from build123d import *

# Parameters (mm, degrees)
EXTRUDE_1_DEPTH     = 10
CUT_EXTRUDE_1_REACH = 177.427
SKETCH_2_R          = 2.15
FILLET_1_R          = 0.6


with BuildPart() as part:
    # 草图1 → 凸台-拉伸1 (new body)
    with BuildSketch(Plane(origin=(0, 0, 0), x_dir=(1, 0, 0), z_dir=(0, 1, 0))):
        with BuildLine():
            Line((-19, 0), (19, 0))
            Line((19, 0), (44.854614973, 30.81233028))
            ThreePointArc((44.854614973, 30.81233028), (46.529317931, 33.929104052), (46.82231051, 37.455159084))
            Line((46.82231051, 37.455159084), (33.389549678, 146.856216784))
            ThreePointArc((33.389549678, 146.856216784), (34.753999407, 148.533855984), (36.376927445, 147.104765038))
            ThreePointArc((36.376927445, 147.104765038), (36.892496808, 144.296291333), (37.320815542, 141.473193853))
            Line((37.320815542, 141.473193853), (37.815132232, 139.258398169))
            ThreePointArc((37.815132232, 139.258398169), (37.817176658, 139.245056143), (37.817405692, 139.231560332))
            Line((37.817405692, 139.231560332), (37.557917484, 134.104765038))
            ThreePointArc((37.557917484, 134.104765038), (40.754926912, 130.959847465), (43.503129215, 134.503681536))
            Line((43.503129215, 134.503681536), (43.077003941, 137.813685213))
            Line((43.077003941, 137.813685213), (42.807637334, 138.925557366))
            ThreePointArc((42.807637334, 138.925557366), (42.806315787, 138.931905108), (42.80540838, 138.938325149))
            Line((42.80540838, 138.938325149), (42.129277547, 145.175318139))
            Line((42.129277547, 145.175318139), (41.965181023, 146.44996701))
            ThreePointArc((41.965181023, 146.44996701), (43.130662006, 148.010841711), (44.727999785, 146.895858405))
            Line((44.727999785, 146.895858405), (66.016482503, 37.376109146))
            ThreePointArc((66.016482503, 37.376109146), (66.063066684, 33.817543133), (64.860464706, 30.468019192))
            Line((64.860464706, 30.468019192), (38.23055697, -15.656334008))
            ThreePointArc((38.23055697, -15.656334008), (35.050772773, -18.836118205), (30.707106781, -20))
            Line((30.707106781, -20), (5.707106781, -20))
            ThreePointArc((5.707106781, -20), (5.515765065, -19.961939766), (5.353553391, -19.853553391))
            Line((5.353553391, -19.853553391), (5, -19.5))
            Line((5, -19.5), (-5, -19.5))
            Line((-5, -19.5), (-5.353553391, -19.853553391))
            ThreePointArc((-5.353553391, -19.853553391), (-5.515765065, -19.961939766), (-5.707106781, -20))
            Line((-5.707106781, -20), (-25.399802658, -20))
            ThreePointArc((-25.399802658, -20), (-30.087775174, -18.833058003), (-33.681629288, -15.604582738))
            Line((-33.681629288, -15.604582738), (-64.860464706, 30.468019192))
            ThreePointArc((-64.860464706, 30.468019192), (-66.063066684, 33.817543133), (-66.016482503, 37.376109146))
            Line((-66.016482503, 37.376109146), (-46.829620455, 141.890886738))
            ThreePointArc((-46.829620455, 141.890886738), (-43.465252598, 152.148967586), (-37.480163066, 161.13372674))
            ThreePointArc((-37.480163066, 161.13372674), (-33.620696298, 161.680216975), (-32.479267504, 157.953116813))
            ThreePointArc((-32.479267504, 157.953116813), (-35.579400499, 146.14570295), (-34.973851142, 133.953116813))
            Line((-34.973851142, 133.953116813), (-47.176674229, 34.569098196))
            ThreePointArc((-47.176674229, 34.569098196), (-47.109221395, 33.75732882), (-46.723670812, 33.03978429))
            Line((-46.723670812, 33.03978429), (-19, 0))
        make_face()
    extrude(amount=EXTRUDE_1_DEPTH)

    # 草图2 → 切除-拉伸1 (cut, up to next)
    with BuildSketch(Plane(origin=(0, 10, 0), x_dir=(1, 0, 0), z_dir=(0, 1, 0)), mode=Mode.PRIVATE) as cut_extrude_1_sk1:
        with Locations(Location((0, -15.5, 0), (0, 0, 270))):
            Circle(SKETCH_2_R)
    cut_extrude_1_tool1 = extrude(cut_extrude_1_sk1.sketch, amount=-CUT_EXTRUDE_1_REACH, mode=Mode.PRIVATE) & part.part
    # 草图2 → 切除-拉伸1 (cut, up to next)
    with BuildSketch(Plane(origin=(0, 10, 0), x_dir=(1, 0, 0), z_dir=(0, 1, 0)), mode=Mode.PRIVATE) as cut_extrude_1_sk2:
        with Locations(Location((0, -7.5, 0), (0, 0, 270))):
            Circle(SKETCH_2_R)
    cut_extrude_1_tool2 = extrude(cut_extrude_1_sk2.sketch, amount=-CUT_EXTRUDE_1_REACH, mode=Mode.PRIVATE) & part.part
    # 草图2 → 切除-拉伸1 (cut, up to next)
    with BuildSketch(Plane(origin=(0, 10, 0), x_dir=(1, 0, 0), z_dir=(0, 1, 0)), mode=Mode.PRIVATE) as cut_extrude_1_sk3:
        with Locations(Location((-26, -10, 0), (0, 0, 270))):
            Circle(SKETCH_2_R)
    cut_extrude_1_tool3 = extrude(cut_extrude_1_sk3.sketch, amount=-CUT_EXTRUDE_1_REACH, mode=Mode.PRIVATE) & part.part
    # 草图2 → 切除-拉伸1 (cut, up to next)
    with BuildSketch(Plane(origin=(0, 10, 0), x_dir=(1, 0, 0), z_dir=(0, 1, 0)), mode=Mode.PRIVATE) as cut_extrude_1_sk4:
        with Locations(Location((26, -10, 0), (0, 0, 270))):
            Circle(SKETCH_2_R)
    cut_extrude_1_tool4 = extrude(cut_extrude_1_sk4.sketch, amount=-CUT_EXTRUDE_1_REACH, mode=Mode.PRIVATE) & part.part
    # 草图2 → 切除-拉伸1 (cut, up to next)
    with BuildSketch(Plane(origin=(0, 10, 0), x_dir=(1, 0, 0), z_dir=(0, 1, 0)), mode=Mode.PRIVATE) as cut_extrude_1_sk5:
        with BuildLine():
            Line((-36.549558395, 121.120011078), (-38.607748185, 104.35740041))
            ThreePointArc((-38.607748185, 104.35740041), (-42.47341142, 116.594845153), (-44.332546284, 129.292956179))
            Line((-44.332546284, 129.292956179), (-43.845113062, 129.987442667))
            ThreePointArc((-43.845113062, 129.987442667), (-43.702378092, 130.509625408), (-43.924830211, 131.003146575))
            Line((-43.924830211, 131.003146575), (-44.447419993, 131.543571067))
            ThreePointArc((-44.447419993, 131.543571067), (-44.482588605, 132.737575539), (-44.499925482, 133.931972015))
            ThreePointArc((-44.499925482, 133.931972015), (-41.418283025, 136.952003662), (-38.505677682, 133.768634142))
            ThreePointArc((-38.505677682, 133.768634142), (-38.556072369, 132.542586282), (-38.556286633, 131.315503182))
            Line((-38.556286633, 131.315503182), (-38.546052546, 131.325051295))
            ThreePointArc((-38.546052546, 131.325051295), (-38.780683801, 130.91622187), (-38.744387532, 130.446247504))
            Line((-38.744387532, 130.446247504), (-38.486748585, 129.793872308))
            ThreePointArc((-38.486748585, 129.793872308), (-37.841140795, 125.384806825), (-36.549558395, 121.120011078))
        make_face()
    cut_extrude_1_tool5 = extrude(cut_extrude_1_sk5.sketch, amount=-CUT_EXTRUDE_1_REACH, mode=Mode.PRIVATE) & part.part
    add(cut_extrude_1_tool1.solids().sort_by_distance((0, 10, 15.5))[0], mode=Mode.SUBTRACT)
    add(cut_extrude_1_tool2.solids().sort_by_distance((0, 10, 7.5))[0], mode=Mode.SUBTRACT)
    add(cut_extrude_1_tool3.solids().sort_by_distance((-26, 10, 10))[0], mode=Mode.SUBTRACT)
    add(cut_extrude_1_tool4.solids().sort_by_distance((26, 10, 10))[0], mode=Mode.SUBTRACT)
    add(cut_extrude_1_tool5.solids().sort_by_distance((-40.502089, 10, -123.156617))[0], mode=Mode.SUBTRACT)

    # 圆角1
    fillet_1_edges = [part.edges().sort_by_distance(p)[0] for p in [
        (-36.549558395, 5, -121.120011078),
        (-34.973851142, 5, -133.953116813),
    ]]
    fillet(fillet_1_edges, radius=FILLET_1_R)


solid = part.part
The listing builds one solid part. Answer for the finished solid, in the listing's coordinates (mm). A direction names the side the tool comes from. Coordinates: 2 decimals unless noted, no trailing zeros. Loops run counter-clockwise (first coordinate to the right, second up) from the corner with the lowest first, then second, coordinate; pieces in that order, holes last. Notation, with made-up numbers: (83.25, 49) -> (108.25, 49) arc R30 ccw to (108.25, 81) -> close; hole circle Ø11 at (58.25, -29). An arc over 180 degrees is marked (long way). Answer in a Markdown table with one row per item. Add a question column.
1. The part is cut by section C-C, the plane y = 4.75. Count the separate pieces of the cut face and the enclosed holes in it, then the cut area to 3 significant figures.
2. The part is cut by section B-B, the plane x = 13. Write down the section's boundary in (y, z), then the cut area to 3 significant figures.
3. Flat-ended cylindrical pins translate along their axes: P1, Ø1.5, axis at y = 5.5, z = -67.5, coming from the +X side; P2, Ø6, axis at x = -40, y = 6, coming from the -Z side; P3, Ø1.5, axis at x = -14.5, y = 5, coming from the -Z side. Find the tip coordinate at first contact, or state that the pin passes through.
4. Consider line 1 (X direction, y = 4.5, z = -37.5); line 2 (Z direction, x = -12.5, y = 8.5); line 3 (X direction, y = 3.25, z = -85). Determine where each line is inside the solid, lowest interval first. Write a range as [from, to].
5. For faces 1 (the flat face through (0, 5, 19.5)), 2 (the cylindrical face through (-38.11, 5.07, -126.74)), 3 (the cylindrical face through (35.11, 4.93, 18.8)), 4 (the flat face through (0, 5, 0)), determine the directions among +Z, -Z, +X, -X, +Y, -Y from which every point of the face is accessible in a straight line to the end or side of a thin tool.
6. Determine the mould class of faces 5 (the flat face through (-15, 5, 20)), 6 (the cylindrical face through (-41.486, 5.07, -136.953)), 7 (the flat face through (51.732, 4.93, -7.729)) for opening direction X: +X half, -X half, draft (parallel to the pull), parting line (faces both ways), or undercut.
7. The part is cut by section A-A, the plane z = -44. Write down the section's boundary in (x, y), then the cut area to 3 significant figures.
Answer below:
| question | item | result |
|---|---|---|
| 1 | separate pieces | 1 |
| 1 | enclosed holes | 4 |
| 1 | area | 6,490 mm2 |
| 2 | outline | (0, 0) -> (10, 0) -> (10, 20) -> (0, 20) -> close |
| 2 | area | 200 mm2 |
| 3 | P1 | x = 60.31 |
| 3 | P2 | z = -161.57 |
| 3 | P3 | z = 0 |
| 4 | line 1 | [-65.99, -46.82], [46.82, 65.99] |
| 4 | line 2 | [0, 20] |
| 4 | line 3 | [-57.27, -40.98], [40.98, 56.76] |
| 5 | face 1 | +Z, +Y, -Y |
| 5 | face 2 | +Y, -Y |
| 5 | face 3 | +Z, +X, +Y, -Y |
| 5 | face 4 | -Z, +Y, -Y |
| 6 | face 5 | draft |
| 6 | face 6 | undercut |
| 6 | face 7 | +X half |
| 7 | outline | (-64.8, 0) -> (-46.02, 0) -> (-46.02, 10) -> (-64.8, 10) -> close; (46.02, 0) -> (64.73, 0) -> (64.73, 10) -> (46.02, 10) -> close |
| 7 | area | 375 mm2 |
